```python
from build123d import *

# Parameters (mm, degrees)
SKETCH_1_W          = 22
SKETCH_1_H          = 3
EXTRUDE_1_DEPTH     = 90
SKETCH_2_W          = 10
SKETCH_2_H          = 10
CUT_EXTRUDE_1_DEPTH = 1


with BuildPart() as part:
    # 草图1 → 凸台-拉伸1 (new body)
    with BuildSketch(Plane.XY):
        with BuildLine():
            Line((0, 4), (22, 4))
            ThreePointArc((22, 4), (22.707106781, 3.707106781), (23, 3))
            Line((23, 3), (23, 0))
            ThreePointArc((23, 0), (22.707106781, -0.707106781), (22, -1))
            Line((22, -1), (0, -1))
            ThreePointArc((0, -1), (-0.707106781, -0.707106781), (-1, 0))
            Line((-1, 0), (-1, 3))
            ThreePointArc((-1, 3), (-0.707106781, 3.707106781), (0, 4))
        make_face()
        with Locations((11, 1.5)):
            Rectangle(SKETCH_1_W, SKETCH_1_H, mode=Mode.SUBTRACT)
    extrude(amount=EXTRUDE_1_DEPTH)

    # 草图2 → 切除-拉伸1 (cut)
    with BuildSketch(Plane(origin=(0, 4, 0), x_dir=(1, 0, 0), z_dir=(0, 1, 0))):
        with Locations((11, -5)):
            Rectangle(SKETCH_2_W, SKETCH_2_H)
    extrude(amount=-CUT_EXTRUDE_1_DEPTH, mode=Mode.SUBTRACT)


solid = part.part
```
Could you check a few things on this model? Use its own coordinates, in mm. A direction names the side the tool comes from. Round coordinates to 2 decimals unless told otherwise and drop trailing zeros. Loops run counter-clockwise (first coordinate to the right, second up) from the corner with the lowest first, then second, coordinate; pieces in that order, holes last. Notation, with made-up numbers: (53, 55) - (103, 55) arc R20 ccw to (103, 92) - close; hole circle Ø9 at (6.5, -8.5). An arc over 180 degrees is marked (long way). Answer in a Markdown table with one row per item. Add a question column.
(1) I'm going to push flat-ended pins straight in: pin 1 (0.5 mm diameter, centred on y = 3.5, z = 3.5, fed in from -X); pin 2 (0.5 mm diameter, centred on x = 9.5, y = 3.5, fed in from -Z); pin 3 (0.8 mm diameter, centred on y = 3.5, z = 7.5, fed in from +X) (3 decimals). Where does each tip first touch, or does it pass through?
(2) If we section it at A-A (x = 3.5): Please give me the cut outline in (y, z), plus the area to 3 significant figures.
(3) For faces 5 (the face through (11, 3, 44)), 6 (the face through (11.2, 3.2, 90)), which set-ups out of +Z, -Z, +X, -X, +Y, -Y let a thin tool reach every point of the face, with its end or its side?
(4) If we mould it in two halves opening along X, with no side actions, what happens to faces 1 (the face through (-1, 1, 44)), 2 (the face through (11, 4, 44)), 3 (the face through (23, 2, 44)), 4 (the face through (11, 0, 44))? For each: pulls with the +X half, pulls with the -X half, needs draft (parallel to the pull), parting line crosses it, or undercut.
(5) If we section it at C-C (z = 67): Please give me the cut outline in (x, y).
(6) If we section it at B-B (y = 2.25): Please give me the cut outline in (x, z).
(7) I need wall thicknesses on line 1 along Y through (x, z) = (16.5, 50.5); line 2 along X through (y, z) = (2.9, 85.5); line 3 along Y through (x, z) = (7.5, 7). Which ranges of each line are inside material? Lowest first, please.
Model answer:
| question | item | result |
|---|---|---|
| 1 | pin 1 | stops at x = -0.97 |
| 1 | pin 2 | stops at z = 10 |
| 1 | pin 3 | stops at x = 22.995 |
| 2 | outline | (-1, 0) - (0, 0) - (0, 90) - (-1, 90) - close; (3, 0) - (4, 0) - (4, 90) - (3, 90) - close |
| 2 | area | 180 mm² |
| 3 | face 5 | +Z, -Z |
| 3 | face 6 | +Z, +X, -X, +Y, -Y |
| 4 | face 1 | pulls with the -X half |
| 4 | face 2 | needs draft |
| 4 | face 3 | pulls with the +X half |
| 4 | face 4 | undercut |
| 5 | outline | (-1, 0) arc R1 ccw to (0, -1) - (22, -1) arc R1 ccw to (23, 0) - (23, 3) arc R1 ccw to (22, 4) - (0, 4) arc R1 ccw to (-1, 3) - close; hole (0, 0) - (22, 0) - (22, 3) - (0, 3) - close |
| 6 | outline | (-1, 0) - (0, 0) - (0, 90) - (-1, 90) - close; (22, 0) - (23, 0) - (23, 90) - (22, 90) - close |
| 7 | line 1 | y = -1 to 0, 3 to 4 |
| 7 | line 2 | x = -1 to 0, 22 to 23 |
| 7 | line 3 | y = -1 to 0 |
